Can you work these out from the drawing? Everything is in mm from the part's minimum corner. A direction names the side the tool comes from. Give positions to 0.01 mm unless a question says otherwise; leave off trailing zeros. Write each loop counter-clockwise with the first axis right and the second up, starting at its lowest first coordinate (ties: lowest second). Pieces come first, ordered by that corner, then holes. Notation, with made-up numbers: (82, 42) - (105, 42) arc R17 ccw to (105, 73) - close; hole circle Ø4 at (-29.5, 18). An arc over 180 degrees is marked (long way). Use a Markdown table: item, result.
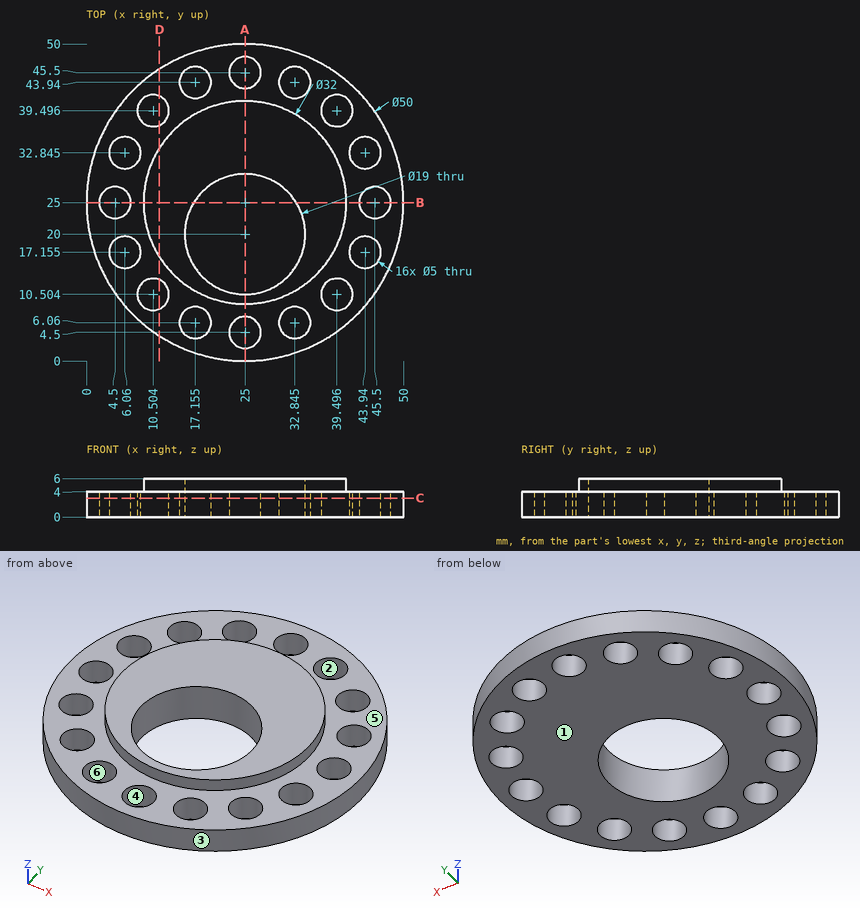
Item 1: Thinking about a two-plate mould opening in X: for the marked faces 1, 2, 3 and 4, which applies, +X half, -X half, draft (parallel to the pull), parting line (faces both ways), or undercut?
Values:
| item | result |
|---|---|
| face 1 | draft |
| face 2 | undercut |
| face 3 | parting line |
| face 4 | undercut |
Item 2: If we section it at C-C, the plane z = 3: Count the separate pieces of the cut face and the enclosed holes in it, plus the area to 3 significant figures.
Values:
| item | result |
|---|---|
| separate pieces | 1 |
| enclosed holes | 17 |
| area | 1,370 mm2 |
Item 3: I need wall thicknesses on line 1 along Y through (x, z) = (25, 0.9); line 2 along Y through (x, z) = (42.5, 2.7) (1 decimal); line 3 along X through (y, z) = (39.5, 0.7) (1 decimal). Which ranges of each line are inside material? Lowest first, please. Write a range as [from, to].
Values:
| item | result |
|---|---|
| line 1 | y = [0, 2], [7, 10.5], [29.5, 43], [48, 50] |
| line 2 | y = [7.1, 15.1], [19.2, 30.8], [34.9, 42.9] |
| line 3 | x = [4.6, 8], [13, 37], [42, 45.4] |
Item 4: If we section it at A-A, the plane x = 25: Write out the boundary of the cut face in (y, z).
Values:
| item | result |
|---|---|
| outline | (0, 0) - (2, 0) - (2, 4) - (0, 4) - close; (7, 0) - (10.5, 0) - (10.5, 6) - (9, 6) - (9, 4) - (7, 4) - close; (29.5, 0) - (43, 0) - (43, 4) - (41, 4) - (41, 6) - (29.5, 6) - close; (48, 0) - (50, 0) - (50, 4) - (48, 4) - close |
Item 5: If we section it at D-D, the plane x = 11.5: Write out the boundary of the cut face in (y, z).
Values:
| item | result |
|---|---|
| outline | (3.96, 0) - (8.21, 0) - (8.21, 4) - (3.96, 4) - close; (12.8, 0) - (37.2, 0) - (37.2, 4) - (33.59, 4) - (33.59, 6) - (16.41, 6) - (16.41, 4) - (12.8, 4) - close; (41.79, 0) - (46.04, 0) - (46.04, 4) - (41.79, 4) - close |
Item 6: For the marked faces 5 and 6, which set-ups out of +Z, -Z, +X, -X, +Y, -Y let a thin tool reach every point of the face, with its end or its side?
Values:
| item | result |
|---|---|
| face 5 | +Z |
| face 6 | +Z, -Z |
Item 7: If we section it at B-B, the plane y = 25: Write out the boundary of the cut face in (x, z), plus the area to 3 significant figures.
Values:
| item | result |
|---|---|
| outline | (0, 0) - (2, 0) - (2, 4) - (0, 4) - close; (7, 0) - (16.92, 0) - (16.92, 6) - (9, 6) - (9, 4) - (7, 4) - close; (33.08, 0) - (43, 0) - (43, 4) - (41, 4) - (41, 6) - (33.08, 6) - close; (48, 0) - (50, 0) - (50, 4) - (48, 4) - close |
| area | 127 mm2 |
Item 8: Will these pins go through, and if not, where does the flat tip stop? pin 1 Ø8 at (x, y) = (6.06, 32.85) entering from +Z; pin 2 Ø15 at (x, y) = (25, 20) entering from +Z; pin 3 Ø2 at (x, z) = (32, 4) entering from +Y.
Values:
| item | result |
|---|---|
| pin 1 | stops at z = 4 |
| pin 2 | passes through |
| pin 3 | stops at y = 49.27 |
